from build123d import *

# Parameters (mm, degrees)
ESQUISSE1_W        = 600
ESQUISSE1_H        = 28
BOSS_EXTRU_1_DEPTH = 28
CONG_1_R           = 28


with BuildPart() as part:
    # Esquisse1 → Boss.-Extru.1 (new body)
    with BuildSketch(Plane.XY):
        with Locations((188.823529412, 32.735294118)):
            Rectangle(ESQUISSE1_W, ESQUISSE1_H)
    extrude(amount=BOSS_EXTRU_1_DEPTH)

    # Congé1
    cong_1_edges = [part.edges().sort_by_distance(p)[0] for p in [
        (188.823529412, 46.735294118, 28),
    ]]
    fillet(cong_1_edges, radius=CONG_1_R - 0.0001)  # a hair under: the kernel refuses the full size


solid = part.part
Here's how the part is built. I have some questions about the finished solid (model axes, mm). Round coordinates to 2 decimals unless told otherwise and drop trailing zeros. Write each loop counter-clockwise with the first axis right and the second up, starting at its lowest first coordinate (ties: lowest second). Pieces come first, ordered by that corner, then holes. Notation, with made-up numbers: (-8, 43) -> (-1, 43) arc R35 ccw to (-1, 80) -> close; hole circle Ø6 at (79.25, -0.5). An arc over 180 degrees is marked (long way). One line per item, written item: value.
1) If I drill on line 1 (Z direction, x = 48, y = 20); line 2 (Z direction, x = 376, y = 44.5); line 3 (Y direction, x = 49, z = 4.5), over which ranges is the centre line in solid material (lowest first)? Write a range as [from, to].
Filled sheet:
line 1: z = [0, 27.97]
line 2: z = [0, 10.96]
line 3: y = [18.74, 46.37]
2) We'd pull the mould along Z, two halves only. Please class faces 1 (the face through (185, 33, 0)), 2 (the face through (193.02, 38.75, 19.58)), 3 (the face through (185, 18.735, 14)): released by +Z, released by -Z, zero draft, split by the parting line, or undercut.
Filled sheet:
face 1: released by -Z
face 2: released by +Z
face 3: zero draft
3) Suppose I cut it at C-C on z = 10. List the corners of the cut face in (x, y) for me.
Filled sheet:
outline: (-111.18, 18.74) -> (488.82, 18.74) -> (488.82, 44.89) -> (-111.18, 44.89) -> close
4) I'm going to push flat-ended pins straight in: pin 1 Ø12 at (x, y) = (326.5, 30.5) entering from +Z; pin 2 Ø6 at (x, z) = (279, 15) entering from +Y. Where does each tip first touch, or does it pass through?
Filled sheet:
pin 1: stops at z = 27.4
pin 2: stops at y = 44.03
5) Suppose I cut it at B-B on y = 40. List the corners of the cut face in (x, z) for me, plus the area to 3 significant figures.
Filled sheet:
outline: (-111.18, 0) -> (488.82, 0) -> (488.82, 18.22) -> (-111.18, 18.22) -> close
area: 10,900 mm2
